Model file for the job. Use its own axes, mm. Face numbers are marked on the shaded views. A direction names the side the tool comes from. Coordinates: 2 decimals unless noted, no trailing zeros. Order: outer loops, then holes, each group sorted by start corner. A loop starts at its lowest first (then second) coordinate and runs counter-clockwise, first axis right, second up. Notation, with made-up numbers: (29, -24.5) -> (65, -24.5) arc R13 ccw to (65, -18.5) -> close; hole circle Ø1 at (-13.5, -26). An arc over 180 degrees is marked (long way). Use CSV: the item, a comma, the result in double quotes. Start each with the question number.
(1) Probe L1, parallel to Y at x = 9, z = 0; L2, parallel to X at y = 9.75, z = -3.75; L3, parallel to X at y = -3.75, z = 3.25. List the from-to ranges inside material, lowest first.
(2) Cut at C-C on x = 12. Write the cut outline in (y, z).
(3) Pin check, flat tips, straight feed: pin 1 Ø7 at (y, z) = (0, 0) entering from +X; pin 2 Ø4 at (y, z) = (9, 0) entering from -X; pin 3 Ø1 at (x, y) = (3.5, -6) entering from -Z; pin 4 Ø3 at (x, y) = (6, 4) entering from -Z. Stop position of each tip, or through.
(4) Tool access for the marked faces 5 and 6: list every direction of +Z, -Z, +X, -X, +Y, -Y with a clear straight run to the whole face (end or side of a thin tool).
(5) Pull direction Y, two halves, no side cores. Call the marked faces 1, 2, 3 and 4: pulls with the +Y half, pulls with the -Y half, needs draft (parallel to the pull), parting line crosses it, or undercut.
(6) Cut at D-D on z = 9. Write the cut outline in (x, y).
(7) Cut at A-A on z = 0. Write the cut outline in (x, y), plus the area to 3 significant figures.
```python
from build123d import *

# Parameters (mm, degrees)
SKETCH1_R           = 6
SKETCH1_R_2         = 4
BOSS_EXTRUDE1_DEPTH = 10
SKETCH2_R           = 12
SKETCH2_R_2         = 1.5
SKETCH2_R_3         = 4
BOSS_EXTRUDE3_DEPTH = 3
SKETCH3_R           = 2
CUT_EXTRUDE1_DEPTH  = 3


with BuildPart() as part:
    # Sketch1 → Boss-Extrude1 (new body)
    with BuildSketch(Plane(origin=(0, 0, 0), x_dir=(0, 0, -1), z_dir=(1, 0, 0))):
        Circle(SKETCH1_R)
        Circle(SKETCH1_R_2, mode=Mode.SUBTRACT)
    extrude(amount=BOSS_EXTRUDE1_DEPTH)

    # Sketch2 → Boss-Extrude3 (add)
    with BuildSketch(Plane(origin=(10, 0, 0), x_dir=(0, 0, -1), z_dir=(1, 0, 0))):
        Circle(SKETCH2_R)
        with Locations((0, 9)):
            Circle(SKETCH2_R_2, mode=Mode.SUBTRACT)
        with Locations((-9, 0)):
            Circle(SKETCH2_R_2, mode=Mode.SUBTRACT)
        with Locations((0, -9)):
            Circle(SKETCH2_R_2, mode=Mode.SUBTRACT)
        with Locations((9, 0)):
            Circle(SKETCH2_R_2, mode=Mode.SUBTRACT)
        Circle(SKETCH2_R_3, mode=Mode.SUBTRACT)
    extrude(amount=BOSS_EXTRUDE3_DEPTH)

    # Sketch3 → Cut-Extrude1 (cut)
    with BuildSketch(Plane(origin=(0, -4.242640687, 4.242640687), x_dir=(-1, 0, 0), z_dir=(0, -0.7071067811865488, 0.7071067811865464))):
        with Locations(Location((-5, 0, 0), (0, 0, 90))):
            Circle(SKETCH3_R)
    extrude(amount=-CUT_EXTRUDE1_DEPTH, mode=Mode.SUBTRACT)


solid = part.part
```
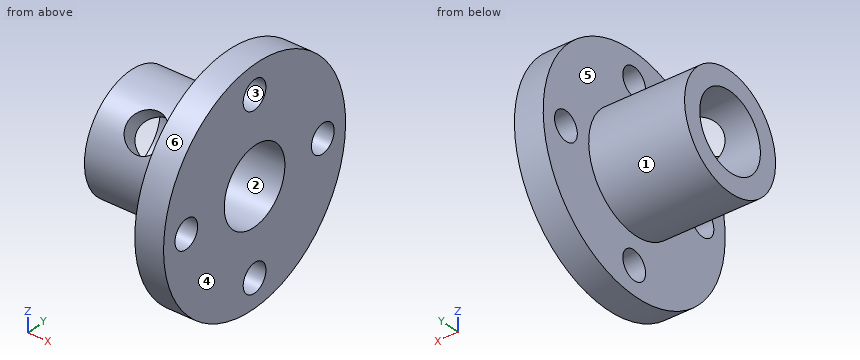
Outcome:
1,L1,"-6 to -4, 4 to 6"
1,L2,"10 to 13"
1,L3,"0 to 3.03, 6.97 to 13"
2,outline,"circle Ø24 at (0, 0); hole circle Ø3 at (-9, 0); hole circle Ø8 at (0, 0); hole circle Ø3 at (0, -9); hole circle Ø3 at (0, 9); hole circle Ø3 at (9, 0)"
3,pin 1,"through"
3,pin 2,"x = 10"
3,pin 3,"z = -2.4"
3,pin 4,"z = -5.45"
4,face 5,"-X"
4,face 6,"+X, -X"
5,face 1,"parting line crosses it"
5,face 2,"undercut"
5,face 3,"undercut"
5,face 4,"needs draft"
6,outline,"(10, -7.94) -> (13, -7.94) -> (13, -1.5) -> (10, -1.5) -> close; (10, 1.5) -> (13, 1.5) -> (13, 7.94) -> (10, 7.94) -> close"
7,outline,"(0, -6) -> (10, -6) -> (10, -7.5) -> (13, -7.5) -> (13, -4) -> (0, -4) -> close; (0, 4) -> (13, 4) -> (13, 7.5) -> (10, 7.5) -> (10, 6) -> (0, 6) -> close; (10, -12) -> (13, -12) -> (13, -10.5) -> (10, -10.5) -> close; (10, 10.5) -> (13, 10.5) -> (13, 12) -> (10, 12) -> close"
7,area,"70.0 mm2"
